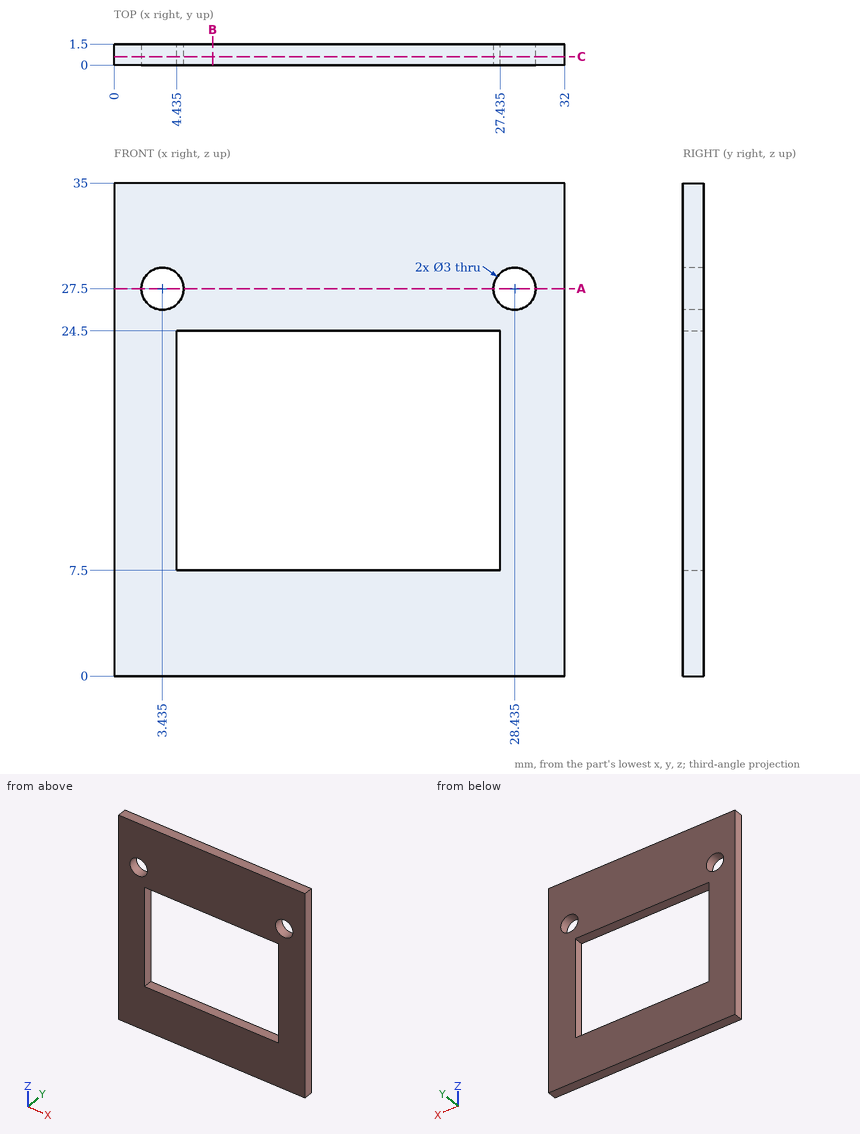
For this review, use the dimensioned drawing (mm, ordinates from the lowest corner) and the shaded views. Coordinates: 2 decimals unless noted, no trailing zeros. Write each loop counter-clockwise with the first axis right and the second up, starting at its lowest first coordinate (ties: lowest second). Pieces come first, ordered by that corner, then holes. Notation, with made-up numbers: (-7.5, 62.25) - (51.5, 62.25) arc R9 cw to (51.5, 74.25) - close; hole circle Ø4 at (-38, -16). An arc over 180 degrees is marked (long way). Answer in a Markdown table with one row per item. Add a question column.
Q1. Consider section B-B on x = 7. Give the boundary of the cut face in (y, z).
Q2. Clearance check with flat-ended pins moving along their axes: pin 1 (1.5 mm diameter, centred on x = 15, z = 10, fed in from -Y); pin 2 (4 mm diameter, centred on x = 3.43, z = 27.5, fed in from -Y). State where each tip first meets the part, or that it passes through.
Q3. Consider section A-A on z = 27.5. Give the boundary of the cut face in (x, y) (3 decimals).
Q4. To check wall thickness, follow line 1 along X through (y, z) = (0.85, 27.5) (3 decimals); line 2 along X through (y, z) = (1, 12.5) (3 decimals); line 3 along Z through (x, y) = (5, 0.45). State the ranges of each line that lie inside material, in increasing order. Write a range as from..to.
Q5. Consider section C-C on y = 0.6. Give the boundary of the cut face in (x, z) (3 decimals), then the cut area to 3 significant figures.
Answers below:
| question | item | result |
|---|---|---|
| 1 | outline | (0, 0) - (1.5, 0) - (1.5, 7.5) - (0, 7.5) - close; (0, 24.5) - (1.5, 24.5) - (1.5, 35) - (0, 35) - close |
| 2 | pin 1 | through |
| 2 | pin 2 | y = 0 |
| 3 | outline | (0, 0) - (1.935, 0) - (1.935, 1.5) - (0, 1.5) - close; (4.935, 0) - (26.935, 0) - (26.935, 1.5) - (4.935, 1.5) - close; (29.935, 0) - (32, 0) - (32, 1.5) - (29.935, 1.5) - close |
| 4 | line 1 | 0..1.935, 4.935..26.935, 29.935..32 |
| 4 | line 2 | 0..4.435, 27.435..32 |
| 4 | line 3 | 0..7.5, 24.5..35 |
| 5 | outline | (0, 0) - (32, 0) - (32, 35) - (0, 35) - close; hole circle Ø3 at (3.435, 27.5); hole (4.435, 7.5) - (27.435, 7.5) - (27.435, 24.5) - (4.435, 24.5) - close; hole circle Ø3 at (28.435, 27.5) |
| 5 | area | 715 mm² |
